```python
from build123d import *

# Parameters (mm, degrees)
F0_W     = 20
F0_H     = 110
F1_DEPTH = 12
F3_DEPTH = 12.001
F4_R     = 5
F5_R     = 5
F6_W     = 9.035658904
F6_H     = 8
F6_W_2   = 2.6605429637
F6_W_3   = 2.1650415125
F7_DEPTH = 110.001


with BuildPart() as f1:
    # F0 (on Top) → F1 (new body)
    with BuildSketch(Plane.XY):
        Rectangle(F0_W, F0_H)
    extrude(amount=F1_DEPTH)

    # F2 (on face) → F3 (cut, through all)
    with BuildSketch(Plane.XY.offset(12)):
        Polygon((6.1587153559, 55), (10, -55), (10, 55), align=None)
        Polygon((-10, 55), (-10, -55), (-6.1587153559, 55), align=None)
    extrude(amount=-F3_DEPTH, mode=Mode.SUBTRACT)

    # F4
    f4_edges = [f1.edges().sort_by_distance(p)[0] for p in [
        (8.079358, 0, 12),
        (10, -55, 6),
        (8.079358, 0, 0),
        (6.158715, 55, 6),
    ]]
    fillet(f4_edges, radius=F4_R)

    # F5
    f5_edges = [f1.edges().sort_by_distance(p)[0] for p in [
        (-10, -55, 6),
        (-8.079358, 0, 12),
        (-6.158715, 55, 6),
        (-8.079358, 0, 0),
    ]]
    fillet(f5_edges, radius=F5_R)

    # F6 (on face) → F7 (cut, through all)
    with BuildSketch(Plane(origin=(0, 55, 0), x_dir=(-1, 0, 0), z_dir=(0, 1, 0))):
        with Locations((-5.8481009339, 6)):
            Rectangle(F6_W, F6_H)
        with Locations((0, 6)):
            Rectangle(F6_W_2, F6_H)
        with Locations((2.4127922381, 6)):
            Rectangle(F6_W_3, F6_H)
    extrude(amount=-F7_DEPTH, mode=Mode.SUBTRACT)


solid = f1.part
```
Read the model definition and answer for the solid it produces. Units are mm, in the model's axes. A direction names the side the tool comes from. Round coordinates to 2 decimals unless told otherwise and drop trailing zeros. Write each loop counter-clockwise with the first axis right and the second up, starting at its lowest first coordinate (ties: lowest second). Pieces come first, ordered by that corner, then holes. Notation, with made-up numbers: (-0.5, 30) - (38.5, 30) arc R15 ccw to (38.5, 38) - close; hole circle Ø1 at (60.5, -15.5). An arc over 180 degrees is marked (long way). One line per item, written item: value.
Q1. For a pull along Z with two mould halves and no side action, classify faces 1 (the flat face through (1, 1, 2)), 2 (the flat face through (1, 1, 10)), 3 (the cylindrical face through (-6.544, 0.894, 1.426)), 4 (the flat face through (-4, -55, 5)) as pulls with the +Z half, pulls with the -Z half, needs draft (parallel to the pull), parting line crosses it, or undercut.
The answers:
face 1: undercut
face 2: undercut
face 3: pulls with the -Z half
face 4: needs draft
Q2. Find section A-A (z = 6). Determine the outline of the cut face in (x, y).
The answers:
outline: (-9.82, -49.83) arc R5 ccw to (-4.82, -55) - (-3.5, -55) - (-3.5, 54.51) arc R5 ccw to (-6.33, 50.17) - close
Q3. Each of these flat-tipped pins is pushed along its axis until it touches: P1, Ø6, axis at y = 28.5, z = 5.5, coming from the -X side; P2, Ø1.5, axis at y = 8.5, z = 5, coming from the +X side; P3, Ø6, axis at x = 7, y = 15, coming from the -Z side. Where does it stop, or does it pass through?
The answers:
P1: stops at x = -7.19
P2: stops at x = -3.5
P3: stops at z = 0.21
Q4. Which of the six approach directions +Z, -Z, +X, -X, +Y, -Y give full straight-line access (tool end or side, diameter ignored) to faces 5 (the flat face through (-3.495, 1, 6)), 6 (the cylindrical face through (5.367, -0.689, 0.542)), 7 (the cylindrical face through (-6.62, 0.9, 10.5)), 8 (the cylindrical face through (5.367, -0.689, 11.458))?
The answers:
face 5: +X, +Y, -Y
face 6: -Z, +X, +Y
face 7: +Z, -X, +Y
face 8: +Z, +X, +Y
Q5. Straight lines are drawn through the part: line 1 (Z direction, x = -1.5, y = 2); line 2 (Z direction, x = 6, y = 13); line 3 (X direction, y = -46, z = 1.25). For each, find the intervals that lie inside material, in ascending order. Write a range as from..to.
The answers:
line 1: z = 0..2, 10..12
line 2: z = 1.31..2, 10..10.69
line 3: x = -7.99..7.99
